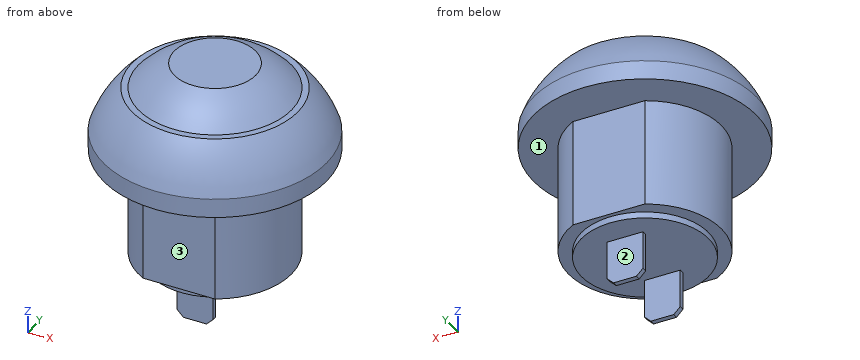
Autodesk Inventor part; units mm, degrees
ref_plane "YZ Plane" through (0, 0, 0) normal (1, 0, 0) x (0, 1, 0)
ref_plane "XZ Plane" through (0, 0, 0) normal (0, 1, 0) x (-1, 0, 0)
ref_plane "XY Plane" through (0, 0, 0) normal (0, 0, 1) x (1, 0, 0)
sketch "Sketch1" plane through (0, 0, 0) normal (0, 1, 0) x (-1, 0, 0)
  line L0 (-8.75, -0.75) -> (8.75, -0.75)
  line L1 (8.75, -0.75) -> (8.75, 0.75)
  line L2 (8.75, 0.75) -> (-8.75, 0.75)
  line L3 (-8.75, 0.75) -> (-8.75, -0.75)
  line L4 (-8.75, -0.75) -> (8.75, 0.75) construction
  line L5 (8.75, -0.75) -> (-8.75, 0.75) construction
  line L6 (6.5, 4.25) -> (-6.5, 4.25)
  line L7 (0, 21.8262) -> (0, -10.0956)
  arc A0 (-6.5, 4.25) -> (-8.75, 0.75) centre (0, -2.4018) ccw
  arc A1 (8.75, 0.75) -> (6.5, 4.25) centre (0, -2.4018) ccw
  line L8 (3.2, 6.25) -> (-3.2, 6.25)
  line L9 (6, 4.25) -> (-6, 4.25)
  arc A2 (6, 4.25) -> (3.2, 6.25) centre (0, -1.19) ccw
  arc A3 (7.8812, 0.6755) -> (7.8632, 0.75) centre (0, -1.19) ccw
  arc A4 (8.087, -0.75) -> (8.0837, -0.6929) centre (0, -1.19) ccw
  arc A5 (-8.0837, -0.6929) -> (-8.087, -0.75) centre (0, -1.19) ccw
  arc A6 (-3.2, 6.25) -> (-6, 4.25) centre (0, -1.19) ccw
  arc A7 (-7.8632, 0.75) -> (-7.8812, 0.6755) centre (0, -1.19) ccw
  line L10 (-6, -9.25) -> (6, -9.25)
  line L11 (6, -9.25) -> (6, -0.75)
  line L12 (6, -0.75) -> (-6, -0.75)
  line L13 (-6, -0.75) -> (-6, -9.25)
  line L14 (-6, -9.25) -> (6, -0.75) construction
  line L15 (6, -9.25) -> (-6, -0.75) construction
  line L16 (-5, -9.75) -> (5, -9.75)
  line L17 (5, -9.75) -> (5, -9.25)
  line L18 (5, -9.25) -> (-5, -9.25)
  line L19 (-5, -9.25) -> (-5, -9.75)
  line L20 (-5, -9.75) -> (5, -9.25) construction
  line L21 (5, -9.75) -> (-5, -9.25) construction
  point P0 (0, 0)
  point P1 (0, 4.25)
  point P2 (0, 0)
  point P3 (0, 6.25)
  point P4 (0, 4.25)
  point P5 (0, -5)
  point P6 (0, -9.5)
  point P7 (0, -9.75)
  dimension "d0" = 17.5
  dimension "d1" = 1.5
  dimension "d2" = 13
  dimension "d3" = 5
  dimension "d4" = 2
  dimension "d5" = 6.4
  dimension "d6" = 12
  dimension "d7" = 12
  dimension "d8" = 8.5
  dimension "d9" = 10
  dimension "d10" = 0.5
revolve "Revolution1" add sketch "Sketch1" angle 360 about axis through (0, 0, 21.8262) along (0, 0, -1) contours L3 L2 L7 L0 | A0 L6 L7 L2 | L0 L7 L10 L13 | A6 L8 L7 L6 | L7 L16 L19 L10
sketch "Sketch2" plane through (0, 0, -9.75) normal (0, 0, -1) x (-1, 0, 0)
  line L0 (0, -14.0708) -> (0, 14.0708) construction
  line L1 (1.4, -2.94) -> (-1.4, -2.94)
  line L2 (-1.4, -2.94) -> (-1.4, -2.54)
  line L3 (-1.4, -2.54) -> (1.4, -2.54)
  line L4 (1.4, -2.54) -> (1.4, -2.94)
  line L5 (1.4, -2.94) -> (-1.4, -2.54) construction
  line L6 (-1.4, -2.94) -> (1.4, -2.54) construction
  line L7 (1.4, 2.94) -> (-1.4, 2.94)
  line L8 (-1.4, 2.94) -> (-1.4, 2.54)
  line L9 (-1.4, 2.54) -> (1.4, 2.54)
  line L10 (1.4, 2.54) -> (1.4, 2.94)
  line L11 (1.4, 2.94) -> (-1.4, 2.54) construction
  line L12 (-1.4, 2.94) -> (1.4, 2.54) construction
  point P0 (0, 0)
  point P1 (0, 0)
  point P2 (0, -2.74)
  point P3 (0, 2.74)
  dimension "d12" = 2.8
  dimension "d13" = 0.4
  dimension "d14" = 2.8
  dimension "d15" = 0.4
  dimension "d16" = 5.08
  dimension "d17" = 2.54
extrude "Extrusion1" add sketch "Sketch2" along normal blind 3.5
chamfer "Chamfer1" distance 0.5 angle 45 4 edges at (1.4, -2.74, -13.25) (-1.4, -2.74, -13.25) (1.4, 2.74, -13.25) (-1.4, 2.74, -13.25)
thread "Thread1"
sketch "Sketch3" plane through (0, 0, -9.25) normal (0, 0, -1) x (-1, 0, 0)
  line L0 (12.7626, -5.3) -> (-12.9759, -5.3)
  line L1 (12.7626, 5.3) -> (-13.4328, 5.3)
  line L2 (14.0115, 0) -> (-13.4328, 0) construction
  circle A0 centre (0, 0) radius 6 construction
  circle A1 centre (0, 0) radius 6
  point P0 (0, 0)
  point P1 (-2.8125, 5.3)
  point P2 (2.8125, 5.3)
  point P3 (-2.8125, -5.3)
  point P4 (2.8125, -5.3)
  dimension "d25" = 10.6
extrude "Extrusion2" cut sketch "Sketch3" against normal up to surface (8.5 mm away) contours A1 L0 | A1 L1
properties part number "Sprung Button DigiKey EG9580-ND"
Can you work these out from the model? Positions are in its coordinate system, mm. Face numbers are marked on the shaded views. A direction names the side the tool comes from. Give positions to 0.01 mm unless a question says otherwise; leave off trailing zeros. Order: outer loops, then holes, each group sorted by start corner. A loop starts at its lowest first (then second) coordinate and runs counter-clockwise, first axis right, second up. Notation, with made-up numbers: M 56,8.25 L 100,8.25 A18 cw 100,43.25 Z; hole C 48,7.5 d6. An arc over 180 degrees is marked long. Use one line per item in the form item = value.
Item 1: If I drill on line 1 along Z through (x, y) = (0, 1.75); line 2 along Y through (x, z) = (-2.75, -2); line 3 along Z through (x, y) = (-4.75, -4), over which ranges is the centre line in solid material (lowest first)? Write a range as [from, to].
Values follow:
line_1 = [-9.75, 6.25]
line_2 = [-5.3, 5.3]
line_3 = [-0.75, 4.25]
Item 2: If we section it at B-B, the plane z = -2: Write out the boundary of the cut face in (x, y), and give its area (3 significant figures).
Values follow:
outline = M -2.81,-5.3 L 2.81,-5.3 A6 ccw 2.81,5.3 L -2.81,5.3 A6 ccw Z
area = 108 mm^2
Item 3: Will these pins go through, and if not, where does the flat tip stop? pin 1 Ø1.7 at (x, z) = (-0.5, -5.5) entering from -Y; pin 2 Ø3 at (x, z) = (-0.5, -12) entering from +Y; pin 3 Ø3 at (x, z) = (0, -12) entering from -Y.
Values follow:
pin_1 = -5.3
pin_2 = 2.94
pin_3 = -2.94
Item 4: For the marked faces 1, 2 and 3, which set-ups out of +Z, -Z, +X, -X, +Y, -Y let a thin tool reach every point of the face, with its end or its side?
Values follow:
face_1 = -Z
face_2 = -Z, +X, -X, +Y
face_3 = -Z, +X, -X, -Y
Item 5: If we section it at C-C, the plane z = 5: Write out the boundary of the cut face in (x, y).
Values follow:
outline = C 0,0 d10.45
Item 6: If we section it at A-A, the plane z = -11.75: Write out the boundary of the cut face in (x, y).
Values follow:
outline = M -1.4,-2.94 L 1.4,-2.94 L 1.4,-2.54 L -1.4,-2.54 Z; M -1.4,2.54 L 1.4,2.54 L 1.4,2.94 L -1.4,2.94 Z
